```python
from build123d import *

# Parameters (mm, degrees)
F0_R     = 3.175
F0_R_2   = 1.5875
F0_R_3   = 6.050143
F0_R_4   = 5.085047
F0_R_5   = 5.029505
F1_DEPTH = 3.048


with BuildPart() as f1:
    # F0 (on Front) → F1 (new body)
    with BuildSketch(Plane.XZ):
        with BuildLine():
            ThreePointArc((-27.6431, 58.259068), (-18.78929, 47.562138), (-8.667807, 57.068443))
            ThreePointArc((-8.667807, 57.068443), (-8.686502, 57.664927), (-8.742514, 58.259068))
            ThreePointArc((-8.742514, 58.259068), (-18.192807, 66.593443), (-27.6431, 58.259068))
        make_face()
        with Locations((-18.192807, 57.068443)):
            Circle(F0_R, mode=Mode.SUBTRACT)
        with BuildLine():
            ThreePointArc((-8.742514, 58.259068), (-8.686502, 57.664927), (-8.667807, 57.068443))
            ThreePointArc((-8.667807, 57.068443), (-18.78929, 47.562138), (-27.6431, 58.259068))
            Line((-27.6431, 58.259068), (-33.943295, 8.252818))
            ThreePointArc((-33.943295, 8.252818), (-18.192807, 22.143443), (-2.442319, 8.252818))
            Line((-2.442319, 8.252818), (-8.742514, 58.259068))
        make_face()
        with Locations((-25.015112, 42.793643)):
            Circle(F0_R_2, mode=Mode.SUBTRACT)
        with BuildLine():
            ThreePointArc((-2.317807, 6.268443), (-2.348966, 7.262582), (-2.442319, 8.252818))
            ThreePointArc((-2.442319, 8.252818), (-18.192807, 22.143443), (-33.943295, 8.252818))
            Line((-33.943295, 8.252818), (-33.29351, 1.371057))
            ThreePointArc((-33.29351, 1.371057), (-16.700506, -9.53626), (-2.442319, 4.284068))
            ThreePointArc((-2.442319, 4.284068), (-2.348966, 5.274305), (-2.317807, 6.268443))
        make_face()
        with Locations((-18.192807, 6.268443)):
            Circle(F0_R_3, mode=Mode.SUBTRACT)
        with BuildLine():
            Line((-33.29351, 1.371057), (-33.943295, 8.252818))
            ThreePointArc((-33.943295, 8.252818), (-33.997511, 4.776142), (-33.29351, 1.371057))
        make_face()
        with BuildLine():
            ThreePointArc((-2.442319, 4.284068), (-16.700506, -9.53626), (-33.29351, 1.371057))
            Line((-33.29351, 1.371057), (-27.675629, -58.126937))
            ThreePointArc((-27.675629, -58.126937), (-18.640994, -47.717107), (-8.667807, -57.231557))
            ThreePointArc((-8.667807, -57.231557), (-11.221517, -63.722068), (-17.513317, -66.732289))
            Line((-17.513317, -66.732289), (26.257193, -65.169057))
            ThreePointArc((26.257193, -65.169057), (18.319693, -57.231557), (26.257193, -49.294057))
            Line((26.257193, -49.294057), (0.772915, -48.383904))
            ThreePointArc((0.772915, -48.383904), (-4.933398, -45.66608), (-6.853743, -39.644382))
            Line((-6.853743, -39.644382), (-2.442319, 4.284068))
        make_face()
        with BuildLine():
            ThreePointArc((-8.667807, -57.231557), (-18.640994, -47.717107), (-27.675629, -58.126937))
            ThreePointArc((-27.675629, -58.126937), (-24.603623, -64.276205), (-18.192807, -66.756557))
            Line((-18.192807, -66.756557), (-17.513317, -66.732289))
            ThreePointArc((-17.513317, -66.732289), (-11.221517, -63.722068), (-8.667807, -57.231557))
        make_face()
        with Locations((-18.192807, -57.231557)):
            Circle(F0_R_4, mode=Mode.SUBTRACT)
        with BuildLine():
            Line((-17.513317, -66.732289), (-18.192807, -66.756557))
            ThreePointArc((-18.192807, -66.756557), (-17.852845, -66.750488), (-17.513317, -66.732289))
        make_face()
        with BuildLine():
            ThreePointArc((34.194693, -57.231557), (31.869853, -51.618897), (26.257193, -49.294057))
            ThreePointArc((26.257193, -49.294057), (18.319693, -57.231557), (26.257193, -65.169057))
            ThreePointArc((26.257193, -65.169057), (31.869853, -62.844217), (34.194693, -57.231557))
        make_face()
        with Locations((26.257193, -57.231557)):
            Circle(F0_R_5, mode=Mode.SUBTRACT)
    extrude(amount=F1_DEPTH)


solid = f1.part
```
Geometry: final body of the model. Coordinates: model frame, mm. A direction names the side the tool comes from. Round coordinates to 2 decimals unless told otherwise and drop trailing zeros. Order: outer loops, then holes, each group sorted by start corner. A loop starts at its lowest first (then second) coordinate and runs counter-clockwise, first axis right, second up. Notation, with made-up numbers: (29.5, 58.5) -> (44.5, 58.5) arc R26 ccw to (44.5, 96.5) -> close; hole circle Ø9 at (58, 23.5). An arc over 180 degrees is marked (long way). Use CSV: the item, a comma, the result in double quotes. Start each with the question number.
1) Draft query along X for faces 3 (the face through (-19.295, -1.503, -62.196)), 4 (the face through (25.167, -1.503, -62.141)), 5 (the face through (-18, -1.5, 66.59)), 6 (the face through (-23, 0, 1)). Return one class per face: +X half, -X half, draft (parallel to the pull), parting line (faces both ways), or undercut.
2) Section A-A (y = -1.3). State how many separate pieces and enclosed holes the cut face has, and give its area (3 significant figures).
3) Material intervals for line 1 along Z through (x, y) = (-20, -2.9); line 2 along X through (y, z) = (-1.65, 6.5); line 3 along X through (y, z) = (-2.05, 58), sorted ascending. Write a range as from..to.
4) Section C-C (x = 9.5). Return the cut outline in (y, z).
5) First-contact query: pin 1 Ø1 at (x, y) = (0.5, -2.5) entering from -Z. Flat tip, straight axial feed; report the tip coordinate or a pass-through.
6) Set-up query: faces 1 (the face through (-30.75, -1.5, 33.61)), 2 (the face through (-4.68, -1.5, -17.99)). Return all of +Z, -Z, +X, -X, +Y, -Y with unobstructed straight access to the full face (end or side cutting, diameter ignored); none if empty.
7) Section B-B (z = 21). Return the cut outline in (x, y), and give its area (3 significant figures).
Returned:
1,face 3,"undercut"
1,face 4,"undercut"
1,face 5,"parting line"
1,face 6,"draft"
2,separate pieces,"1"
2,enclosed holes,"5"
2,area,"3,610 mm²"
3,line 1,"z = -66.58..-61.98, -52.48..0.49, 12.04..54.46, 59.68..66.42"
3,line 2,"x = -34.07..-24.24, -12.15..-2.32"
3,line 3,"x = -27.68..-21.23, -15.16..-8.71"
4,outline,"(-3.05, -65.77) -> (0, -65.77) -> (0, -48.7) -> (-3.05, -48.7) -> close"
5,pin 1,"stops at z = -66.11"
6,face 1,"+Z, -X, +Y, -Y"
6,face 2,"+X, +Y, -Y"
7,outline,"(-32.34, -3.05) -> (-4.05, -3.05) -> (-4.05, 0) -> (-32.34, 0) -> close"
7,area,"86.2 mm²"
